```python
from build123d import *

# Parameters (mm, degrees)
SKETCH1_R           = 44.45
SKETCH1_R_2         = 3
BOSS_EXTRUDE1_DEPTH = 3.81
FILLET1_R           = 2
FILLET2_R           = 2
SKETCH3_R           = 1.5875


with BuildPart() as part:
    # Sketch1 → Boss-Extrude1 (new body)
    with BuildSketch(Plane.XY):
        Circle(SKETCH1_R)
        Circle(SKETCH1_R_2, mode=Mode.SUBTRACT)
        with BuildLine():
            Line((7.52236, -3.452121223), (35.063651683, -5.861672024))
            ThreePointArc((35.063651683, -5.861672024), (25.137808857, -25.137808857), (5.861672024, -35.063651683))
            Line((5.861672024, -35.063651683), (3.452121223, -7.52236))
            ThreePointArc((3.452121223, -7.52236), (5.852479855, -5.852479855), (7.52236, -3.452121223))
        make_face(mode=Mode.SUBTRACT)
        with BuildLine():
            Line((3.452121223, 7.52236), (5.861672024, 35.063651683))
            ThreePointArc((5.861672024, 35.063651683), (25.137808857, 25.137808857), (35.063651683, 5.861672024))
            Line((35.063651683, 5.861672024), (7.52236, 3.452121223))
            ThreePointArc((7.52236, 3.452121223), (5.852479855, 5.852479855), (3.452121223, 7.52236))
        make_face(mode=Mode.SUBTRACT)
        with BuildLine():
            Line((-3.452121223, 7.52236), (-5.861672024, 35.063651683))
            ThreePointArc((-5.861672024, 35.063651683), (-25.137808857, 25.137808857), (-35.063651683, 5.861672024))
            Line((-35.063651683, 5.861672024), (-7.52236, 3.452121223))
            ThreePointArc((-7.52236, 3.452121223), (-5.852479855, 5.852479855), (-3.452121223, 7.52236))
        make_face(mode=Mode.SUBTRACT)
        with BuildLine():
            Line((-3.452121223, -7.52236), (-5.861672024, -35.063651683))
            ThreePointArc((-5.861672024, -35.063651683), (-25.137808857, -25.137808857), (-35.063651683, -5.861672024))
            Line((-35.063651683, -5.861672024), (-7.52236, -3.452121223))
            ThreePointArc((-7.52236, -3.452121223), (-5.852479855, -5.852479855), (-3.452121223, -7.52236))
        make_face(mode=Mode.SUBTRACT)
    extrude(amount=BOSS_EXTRUDE1_DEPTH)

    # Fillet1
    fillet1_edges = [part.edges().sort_by_distance(p)[0] for p in [
        (35.063651683, -5.861672024, 1.905),
        (35.063651683, 5.861672024, 1.905),
    ]]
    fillet(fillet1_edges, radius=FILLET1_R)

    # Fillet2
    fillet2_edges = [part.edges().sort_by_distance(p)[0] for p in [
        (5.861672024, -35.063651683, 1.905),
        (-35.063651683, -5.861672024, 1.905),
        (-5.861672024, -35.063651683, 1.905),
        (5.861672024, 35.063651683, 1.905),
        (-5.861672024, 35.063651683, 1.905),
        (-35.063651683, 5.861672024, 1.905),
    ]]
    fillet(fillet2_edges, radius=FILLET2_R)

    # Sketch3 → Cut-Revolve1 (revolve, cut)
    with BuildSketch(Plane(origin=(0, 0, 0), x_dir=(1, 0, 0), z_dir=(0, 1, 0))):
        with Locations((-44.45, -1.905)):
            Circle(SKETCH3_R)
    revolve(axis=Axis((0, 0, 0), (0, 0, 1)), mode=Mode.SUBTRACT)


solid = part.part
```
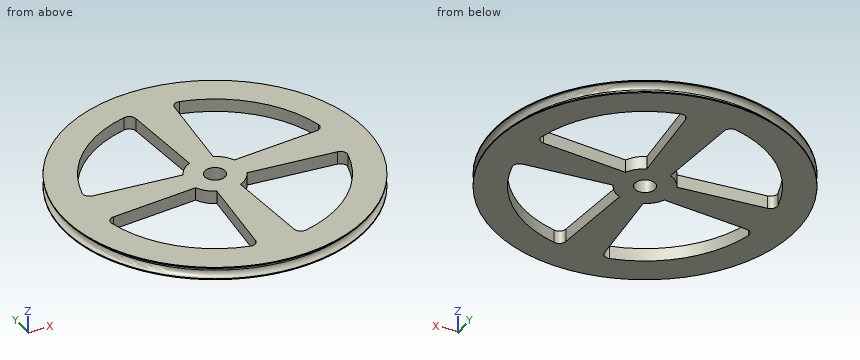
The model under review builds one solid part; all positions refer to its coordinate system, in mm. Coordinates: 2 decimals unless noted, no trailing zeros. Answer in a Markdown table with one row per item. Add a question column.
Item 1: We need section C-C on x = -17. Give the number of separate pieces and of enclosed holes in the cut face, plus the area to 3 significant figures.
Item 2: Clearance check with flat-ended pins moving along their axes: pin 1 (1 mm diameter, centred on y = 0, z = 1, fed in from -X); pin 2 (1 mm diameter, centred on x = -22, z = 0.5, fed in from +Y). State where each tip first meets the part, or that it passes through.
Item 3: To check wall thickness, follow probe 1 along X at (y, z) = (-17.5, 1.15); probe 2 along Y at (x, z) = (-23.5, 1.45); probe 3 along Y at (x, z) = (7, 0.9). State the ranges of each line that lie inside material, in increasing order.
Final values:
| question | item | result |
|---|---|---|
| 1 | separate pieces | 3 |
| 1 | enclosed holes | 0 |
| 1 | area | 99.1 mm2 |
| 2 | pin 1 | stops at x = -43.71 |
| 2 | pin 2 | stops at y = 38.89 |
| 3 | probe 1 | x = -39.34 to -30.94, -4.33 to 4.33, 30.94 to 39.34 |
| 3 | probe 2 | y = -35.93 to -26.68, -4.85 to 4.85, 26.68 to 35.93 |
| 3 | probe 3 | y = -42.65 to -34.55, -4.42 to 4.42, 34.55 to 42.65 |
